from build123d import *

# Parameters (mm, degrees)
F0_R     = 11.2
F0_R_2   = 11
F1_DEPTH = 7
F3_DEPTH = 6.8


with BuildPart() as f1:
    # F0 (on Top) → F1 (new body)
    with BuildSketch(Plane.XY):
        with BuildLine():
            Line((-12.6559794838, 49.3346591402), (-11.0453985259, 47.7240781823))
            ThreePointArc((-11.0453985259, 47.7240781823), (-14.0378256841, 40.9399649675), (-13.2027236571, 33.572372619))
            Line((-13.2027236571, 33.572372619), (-35.6758893819, -5.3522922233))
            ThreePointArc((-35.6758893819, -5.3522922233), (-42.473962534, -8.3128688274), (-46.852963341, -14.2964433728))
            Line((-46.852963341, -14.2964433728), (-49.0530578444, -13.7069298274))
            Line((-49.0530578444, -13.7069298274), (-49.6863089117, -16.6430792565))
            Line((-49.6863089117, -16.6430792565), (-47.6294204763, -17.1942208517))
            ThreePointArc((-47.6294204763, -17.1942208517), (-47.7713823768, -18.4712755649), (-47.7973240691, -19.7559346444))
            Line((-47.7973240691, -19.7559346444), (-50.0555434173, -20.0532348617))
            Line((-50.0555434173, -20.0532348617), (-49.5169753758, -23.0082179156))
            Line((-49.5169753758, -23.0082179156), (-47.4057454924, -22.7302692285))
            ThreePointArc((-47.4057454924, -22.7302692285), (-47.0481935057, -23.9644404073), (-46.5805427582, -25.1612380929))
            Line((-46.5805427582, -25.1612380929), (-48.5530935264, -26.3000908099))
            Line((-48.5530935264, -26.3000908099), (-46.9246984783, -28.8240381057))
            Line((-46.9246984783, -28.8240381057), (-45.0805427582, -27.7593143042))
            ThreePointArc((-45.0805427582, -27.7593143042), (-44.277910933, -28.7627105744), (-43.3878633329, -29.6894452675))
            Line((-43.3878633329, -29.6894452675), (-44.6841888987, -31.3788496362))
            Line((-44.6841888987, -31.3788496362), (-42.3943825269, -33.3227547688))
            Line((-42.3943825269, -33.3227547688), (-41.0078033121, -31.5157295545))
            ThreePointArc((-41.0078033121, -31.5157295545), (-39.8822850679, -32.1355929298), (-38.705342294, -32.6511776742))
            Line((-38.705342294, -32.6511776742), (-39.2564838892, -34.7080661095))
            Line((-39.2564838892, -34.7080661095), (-36.3970783606, -35.6277293129))
            Line((-36.3970783606, -35.6277293129), (-35.8075648151, -33.4276348095))
            ThreePointArc((-35.8075648151, -33.4276348095), (-28.4361368498, -32.6270961401), (-22.4731657248, -28.2200803957))
            Line((-22.4731657248, -28.2200803957), (22.4731657248, -28.2200803957))
            ThreePointArc((22.4731657248, -28.2200803957), (28.4361368498, -32.6270961401), (35.8075648151, -33.4276348095))
            Line((35.8075648151, -33.4276348095), (36.3970783606, -35.6277293129))
            Line((36.3970783606, -35.6277293129), (39.2564838892, -34.7080661095))
            Line((39.2564838892, -34.7080661095), (38.705342294, -32.6511776742))
            ThreePointArc((38.705342294, -32.6511776742), (39.8822850679, -32.1355929298), (41.0078033121, -31.5157295545))
            Line((41.0078033121, -31.5157295545), (42.3943825269, -33.3227547688))
            Line((42.3943825269, -33.3227547688), (44.6841888987, -31.3788496362))
            Line((44.6841888987, -31.3788496362), (43.3878633329, -29.6894452675))
            ThreePointArc((43.3878633329, -29.6894452675), (44.277910933, -28.7627105744), (45.0805427582, -27.7593143042))
            Line((45.0805427582, -27.7593143042), (47.0530935264, -28.8981670212))
            Line((47.0530935264, -28.8981670212), (48.4246984783, -26.2259618943))
            Line((48.4246984783, -26.2259618943), (46.5805427582, -25.1612380929))
            ThreePointArc((46.5805427582, -25.1612380929), (47.0481935057, -23.9644404073), (47.4057454924, -22.7302692285))
            Line((47.4057454924, -22.7302692285), (49.5169753758, -23.0082179156))
            Line((49.5169753758, -23.0082179156), (50.0555434173, -20.0532348617))
            Line((50.0555434173, -20.0532348617), (47.7973240691, -19.7559346444))
            ThreePointArc((47.7973240691, -19.7559346444), (47.7713823768, -18.4712755649), (47.6294204763, -17.1942208517))
            Line((47.6294204763, -17.1942208517), (49.6863089117, -16.6430792565))
            Line((49.6863089117, -16.6430792565), (49.0530578444, -13.7069298274))
            Line((49.0530578444, -13.7069298274), (46.852963341, -14.2964433728))
            ThreePointArc((46.852963341, -14.2964433728), (42.473962534, -8.3128688274), (35.6758893819, -5.3522922233))
            Line((35.6758893819, -5.3522922233), (13.2027236571, 33.572372619))
            ThreePointArc((13.2027236571, 33.572372619), (14.0378256841, 40.9399649675), (11.0453985259, 47.7240781823))
            Line((11.0453985259, 47.7240781823), (12.6559794838, 49.3346591402))
            Line((12.6559794838, 49.3346591402), (10.4298250225, 51.3511453661))
            Line((10.4298250225, 51.3511453661), (8.9240781823, 49.8453985259))
            ThreePointArc((8.9240781823, 49.8453985259), (7.8890973089, 50.6068684947), (6.789520757, 51.2716641989))
            Line((6.789520757, 51.2716641989), (7.6611608904, 53.3759896304))
            Line((7.6611608904, 53.3759896304), (4.8327864772, 54.3870675519))
            Line((4.8327864772, 54.3870675519), (4.0178821595, 52.419714496))
            ThreePointArc((4.0178821595, 52.419714496), (2.7702825726, 52.7271509817), (1.5, 52.9205523971))
            Line((1.5, 52.9205523971), (1.5, 55.1982578311))
            Line((1.5, 55.1982578311), (-1.5, 55.05))
            Line((-1.5, 55.05), (-1.5, 52.9205523971))
            ThreePointArc((-1.5, 52.9205523971), (-2.7702825726, 52.7271509817), (-4.0178821595, 52.419714496))
            Line((-4.0178821595, 52.419714496), (-4.8327864772, 54.3870675519))
            Line((-4.8327864772, 54.3870675519), (-7.6611608904, 53.3759896304))
            Line((-7.6611608904, 53.3759896304), (-6.789520757, 51.2716641989))
            ThreePointArc((-6.789520757, 51.2716641989), (-7.8890973089, 50.6068684947), (-8.9240781823, 49.8453985259))
            Line((-8.9240781823, 49.8453985259), (-10.4298250225, 51.3511453661))
            Line((-10.4298250225, 51.3511453661), (-12.6559794838, 49.3346591402))
        make_face()
        with Locations((-33.6017856668, -19.4)):
            Circle(F0_R, mode=Mode.SUBTRACT)
        Polygon((-12.1033156734, -25.2200803957), (0.172366893, -16.0264908435), (12.1033156734, -25.2200803957), align=None, mode=Mode.SUBTRACT)
        with BuildLine():
            Line((-20.4268113342, -14.1028260993), (-11, -8.6602540378))
            ThreePointArc((-11, -8.6602540378), (-7.0988974128, -12.0667168494), (-2.2263110665, -13.8218500583))
            Line((-2.2263110665, -13.8218500583), (-17.0183247375, -25.2200803957))
            Line((-17.0183247375, -25.2200803957), (-20.649308522, -25.2200803957))
            ThreePointArc((-20.649308522, -25.2200803957), (-19.4046286997, -19.6841373792), (-20.4268113342, -14.1028260993))
        make_face(mode=Mode.SUBTRACT)
        with BuildLine():
            ThreePointArc((-13.0832288111, 4.9828830888), (-13.9995320382, -0.1144670736), (-13, -5.1961524227))
            Line((-13, -5.1961524227), (-22.4268113342, -10.6387244841))
            ThreePointArc((-22.4268113342, -10.6387244841), (-26.7492773718, -6.9628327153), (-32.1658845691, -5.2727855528))
            Line((-32.1658845691, -5.2727855528), (-30.3503926769, -2.1282613547))
            Line((-30.3503926769, -2.1282613547), (-13.0832288111, 4.9828830888))
        make_face(mode=Mode.SUBTRACT)
        with BuildLine():
            ThreePointArc((2.2263110665, -13.8218500583), (7.0988974128, -12.0667168494), (11, -8.6602540378))
            Line((11, -8.6602540378), (20.4268113342, -14.1028260993))
            ThreePointArc((20.4268113342, -14.1028260993), (19.4046286997, -19.6841373792), (20.649308522, -25.2200803957))
            Line((20.649308522, -25.2200803957), (17.0183247375, -25.2200803957))
            Line((17.0183247375, -25.2200803957), (2.2263110665, -13.8218500583))
        make_face(mode=Mode.SUBTRACT)
        with Locations((33.6017856668, -19.4)):
            Circle(F0_R, mode=Mode.SUBTRACT)
        with BuildLine():
            Line((22.4268113342, -10.6387244841), (13, -5.1961524227))
            ThreePointArc((13, -5.1961524227), (13.9995320382, -0.1144670736), (13.0832288111, 4.9828830888))
            Line((13.0832288111, 4.9828830888), (30.3503926769, -2.1282613547))
            Line((30.3503926769, -2.1282613547), (32.1658845691, -5.2727855528))
            ThreePointArc((32.1658845691, -5.2727855528), (26.7492773718, -6.9628327153), (22.4268113342, -10.6387244841))
        make_face(mode=Mode.SUBTRACT)
        Circle(F0_R_2, mode=Mode.SUBTRACT)
        Polygon((-15.7895724715, 23.091819041), (-13.9655316505, 7.8639713136), (-27.8928881448, 2.1282613547), align=None, mode=Mode.SUBTRACT)
        with BuildLine():
            Line((-2, 24.7415505834), (-2, 13.8564064606))
            ThreePointArc((-2, 13.8564064606), (-6.9006346255, 12.181183923), (-10.8569177445, 8.8389669695))
            Line((-10.8569177445, 8.8389669695), (-13.3320679394, 27.3483417504))
            Line((-13.3320679394, 27.3483417504), (-11.5165760472, 30.4928659485))
            ThreePointArc((-11.5165760472, 30.4928659485), (-7.3446486721, 26.6469700945), (-2, 24.7415505834))
        make_face(mode=Mode.SUBTRACT)
        with BuildLine():
            ThreePointArc((10.8569177445, 8.8389669695), (6.9006346255, 12.181183923), (2, 13.8564064606))
            Line((2, 13.8564064606), (2, 24.7415505834))
            ThreePointArc((2, 24.7415505834), (7.3446486721, 26.6469700945), (11.5165760472, 30.4928659485))
            Line((11.5165760472, 30.4928659485), (13.3320679394, 27.3483417504))
            Line((13.3320679394, 27.3483417504), (10.8569177445, 8.8389669695))
        make_face(mode=Mode.SUBTRACT)
        Polygon((27.8928881448, 2.1282613547), (13.7931647575, 8.1625195299), (15.7895724715, 23.091819041), align=None, mode=Mode.SUBTRACT)
        with Locations((0, 38.8)):
            Circle(F0_R, mode=Mode.SUBTRACT)
    extrude(amount=F1_DEPTH)

    # F2 (on face) → F3 (join)
    with BuildSketch(Plane.XY.offset(7)):
        Polygon((27.8928881448, 2.1282613547), (15.7895724715, 23.091819041), (13.7931647575, 8.1625195299), align=None)
        Polygon((-12.1033156734, -25.2200803957), (12.1033156734, -25.2200803957), (0.172366893, -16.0264908435), (-11.5165760472, -24.7806552747), align=None)
        Polygon((-13.9655316505, 7.8639713136), (-15.7895724715, 23.091819041), (-27.8928881448, 2.1282613547), align=None)
    extrude(amount=-F3_DEPTH)


solid = f1.part
Geometry check sheet. Reference: the model listing, model coordinates, mm. A direction names the side the tool comes from. Round coordinates to 2 decimals unless told otherwise and drop trailing zeros. Write each loop counter-clockwise with the first axis right and the second up, starting at its lowest first coordinate (ties: lowest second). Pieces come first, ordered by that corner, then holes. Notation, with made-up numbers: (82, 82.25) -> (139, 82.25) arc R11 ccw to (139, 101.25) -> close; hole circle Ø1 at (-12, -10). An arc over 180 degrees is marked (long way). One line per item, written item: value. Start each with the question number.
(1) Cross-section at B-B, the plane y = 0. Record the cut outline in (x, z).
(2) Go/stop test with flat-tipped pins: pin 1 Ø3 at (y, z) = (19.5, 1.5) entering from -X; pin 2 Ø2 at (x, z) = (-20, 4) entering from +Y; pin 3 Ø1.1 at (x, z) = (-19.5, 3) entering from +Y; pin 4 Ø13 at (x, y) = (0, 0) entering from +Z. Record where each tip stops, or that it passes through.
(3) Access from +Z, -Z, +X, -X, +Y, -Y to the whole of each face (thin tool, end or side, straight path). Record for faces 5 (the cylindrical face through (-2.75, 52.73, 3.45)), 6 (the flat face through (12.11, 18.22, 3.45)), 7 (the flat face through (49.782, -21.551, 3.451)).
(4) Scan lines: line 1 (X direction, y = 38.5, z = 5.75); line 2 (X direction, y = 19, z = 4.5); line 3 (Y direction, x = 14.5, z = 1.5). Record each from-to range of solid material in increasing order. Write a range as [from, to].
(5) Cross-section at D-D, the plane z = 5. Give the number of separate pieces and of enclosed holes in the cut face, and give its area (3 significant figures).
(6) Cross-section at A-A, the plane y = 38.8. Record the cut outline in (x, z), and give its area (3 significant figures).
(7) Draft check along Y on faces 1 (the flat face through (-47.938, -14.006, 3.451)), 2 (the cylindrical face through (14.053, 40.836, 3.451)), 3 (the flat face through (-48.9, -19.9, 3.5)), 4 (the flat face through (11, -3, 0)). Enter one of: +Y half, -Y half, draft (parallel to the pull), parting line (faces both ways), or undercut.
(8) Cross-section at C-C, the plane y = 16.5. Record the cut outline in (x, z).
Answer:
1. outline: (-32.59, 0) -> (-25.18, 0) -> (-25.18, 7) -> (-32.59, 7) -> close; (-14, 0) -> (-11, 0) -> (-11, 7) -> (-14, 7) -> close; (11, 0) -> (14, 0) -> (14, 7) -> (11, 7) -> close; (25.18, 0) -> (32.59, 0) -> (32.59, 7) -> (25.18, 7) -> close
2. pin 1: x = -22.19
2. pin 2: y = 23.53
2. pin 3: y = 23.62
2. pin 4: through
3. face 5: +Z, -Z, +Y
3. face 6: +Z, -Z
3. face 7: +Z, -Z, +X, -Y
4. line 1: [-14.2, -11.2], [11.2, 14.2]
4. line 2: [-21.62, -12.22], [-2, 2], [12.22, 21.62]
4. line 3: [-28.22, -23.28], [-10.68, -6.06], [4.4, 31.33]
5. separate pieces: 1
5. enclosed holes: 10
5. area: 2,220 mm²
6. outline: (-14.2, 0) -> (-11.2, 0) -> (-11.2, 7) -> (-14.2, 7) -> close; (11.2, 0) -> (14.2, 0) -> (14.2, 7) -> (11.2, 7) -> close
6. area: 42.0 mm²
7. face 1: +Y half
7. face 2: undercut
7. face 3: undercut
7. face 4: draft
8. outline: (-23.06, 0) -> (-19.6, 0) -> (-19.6, 0.2) -> (-15, 0.2) -> (-15, 0) -> (-11.88, 0) -> (-11.88, 7) -> (-23.06, 7) -> close; (-2, 0) -> (2, 0) -> (2, 7) -> (-2, 7) -> close; (11.88, 0) -> (14.91, 0) -> (14.91, 0.2) -> (19.6, 0.2) -> (19.6, 0) -> (23.06, 0) -> (23.06, 7) -> (11.88, 7) -> close
